The model under review builds one solid part; all positions refer to its coordinate system, in mm. A direction names the side the tool comes from. Coordinates: 2 decimals unless noted, no trailing zeros. Loops run counter-clockwise (first coordinate to the right, second up) from the corner with the lowest first, then second, coordinate; pieces in that order, holes last. Notation, with made-up numbers: M 61.25,72 L 87.25,72 A23 ccw 87.25,111 Z; hole C -39,2 d7. An arc over 180 degrees is marked long. Use CSV: the item, a comma, the result in double quotes. Start each with the question number.
from build123d import *

# Parameters (mm, degrees)
SKETCH1_R               = 15
SKETCH1_R_2             = 1
BOSS_EXTRUDE1_DEPTH     = 32.6375
SKETCH2_W               = 21.5
SKETCH2_H               = 6.35
CUT_EXTRUDE1_DEPTH      = 16
CUT_EXTRUDE1_DEPTH_BACK = 16
SKETCH3_R               = 1.5
SKETCH3_R_2             = 1
BOSS_EXTRUDE2_DEPTH     = 0.5
SKETCH4_R               = 10
SKETCH4_R_2             = 1
BOSS_EXTRUDE3_DEPTH     = 2.5
CUT_SWEEP2_PROFILE_R    = 1
SKETCH82_R              = 1.5
SKETCH82_R_2            = 1
BOSS_EXTRUDE5_DEPTH     = 0.5
SKETCH91_R              = 15
SKETCH91_R_2            = 8
CUT_EXTRUDE2_DEPTH      = 1.5
CUT_EXTRUDE2_DEPTH_BACK = 8.14375
SKETCH92_R              = 15
SKETCH92_R_2            = 10
CUT_EXTRUDE3_DEPTH      = 8.14375


with BuildPart() as part:
    # Sketch1 → Boss-Extrude1 (new body)
    with BuildSketch(Plane(origin=(0, 0, 0), x_dir=(1, 0, 0), z_dir=(0, 1, 0))):
        Circle(SKETCH1_R)
        Circle(SKETCH1_R_2, mode=Mode.SUBTRACT)
    extrude(amount=BOSS_EXTRUDE1_DEPTH)

    # Sketch2 → Cut-Extrude1 (cut, two sides)
    with BuildSketch(Plane.XY) as cut_extrude1_sk:
        with Locations((0, 16.31875)):
            Rectangle(SKETCH2_W, SKETCH2_H)
    extrude(amount=CUT_EXTRUDE1_DEPTH, mode=Mode.SUBTRACT)
    extrude(cut_extrude1_sk.sketch, amount=-CUT_EXTRUDE1_DEPTH_BACK, mode=Mode.SUBTRACT)

    # Sketch3 → Boss-Extrude2 (add)
    with BuildSketch(Plane(origin=(0, 0, 0), x_dir=(-1, 0, 0), z_dir=(0, -1, 0))):
        Circle(SKETCH3_R)
        Circle(SKETCH3_R_2, mode=Mode.SUBTRACT)
    extrude(amount=BOSS_EXTRUDE2_DEPTH)

    # Sketch4 → Boss-Extrude3 (add)
    with BuildSketch(Plane(origin=(0, 32.6375, 0), x_dir=(1, 0, 0), z_dir=(0, 1, 0))):
        Circle(SKETCH4_R)
        Circle(SKETCH4_R_2, mode=Mode.SUBTRACT)
    extrude(amount=BOSS_EXTRUDE3_DEPTH)

    # Cut-Sweep2: sweep along a path in Sketch77
    with BuildLine(Plane(origin=(0, 33.8875, 0), x_dir=(1, 0, 0), z_dir=(0, 1, 0))) as cut_sweep2_path:
        CenterArc((0, 0), 10, 0, 360)
    # Cut-Sweep2 profile (on start of the path) → Cut-Sweep2 (sweep, cut)
    with BuildSketch(Plane(origin=(10, 33.8875, 0), x_dir=(-1, 0, 0), z_dir=(0, 0, -1))):
        Circle(CUT_SWEEP2_PROFILE_R)
    sweep(path=cut_sweep2_path.line, mode=Mode.SUBTRACT)

    # Sketch82 → Boss-Extrude5 (add)
    with BuildSketch(Plane(origin=(0, 35.1375, 0), x_dir=(1, 0, 0), z_dir=(0, 1, 0))):
        Circle(SKETCH82_R)
        Circle(SKETCH82_R_2, mode=Mode.SUBTRACT)
    extrude(amount=BOSS_EXTRUDE5_DEPTH)

    # Sketch91 → Cut-Extrude2 (cut, two sides)
    with BuildSketch(Plane.XZ) as cut_extrude2_sk:
        Circle(SKETCH91_R)
        Circle(SKETCH91_R_2, mode=Mode.SUBTRACT)
    extrude(amount=CUT_EXTRUDE2_DEPTH, mode=Mode.SUBTRACT)
    extrude(cut_extrude2_sk.sketch, amount=-CUT_EXTRUDE2_DEPTH_BACK, mode=Mode.SUBTRACT)

    # Sketch92 → Cut-Extrude3 (cut)
    with BuildSketch(Plane(origin=(0, 32.6375, 0), x_dir=(1, 0, 0), z_dir=(0, 1, 0))):
        Circle(SKETCH92_R)
        Circle(SKETCH92_R_2, mode=Mode.SUBTRACT)
    extrude(amount=-CUT_EXTRUDE3_DEPTH, mode=Mode.SUBTRACT)


solid = part.part
1. Insertion check: pin 1 Ø13 at (x, z) = (-1.5, 2.5) entering from -Y; pin 2 Ø3 at (x, y) = (11.5, 11) entering from -Z; pin 3 Ø4 at (y, z) = (27.5, -2) entering from -X; pin 4 Ø8 at (x, z) = (0, 7) entering from +Y. Each pin has a flat end and moves straight along its axis. Give the tip position at first contact, or say it passes through.
2. To check wall thickness, follow line 1 along X through (y, z) = (-0.4, 0); line 2 along Y through (x, z) = (-5, -2.75); line 3 along Z through (x, y) = (0, 23.5). State the ranges of each line that lie inside material, in increasing order.
3. Add section B-B (y = 24). Write out the cut boundary in (x, z), plus the area to 3 significant figures.
4. Add section C-C (x = 0). Give the number of separate pieces and of enclosed holes in the cut face, plus the area to 3 significant figures.
5. For faces 1 (the flat face through (6, 8.144, -6)), 2 (the flat face through (-10.75, 16, 0)), 3 (the cylindrical face through (0, 27, 1)), 4 (the flat face through (3, 24.494, 10)), list the 3-axis set-ups (+Z, -Z, +X, -X, +Y, -Y) from which the entire face can be reached by the end or side of a thin tool; tool diameter is ignored.
6. Draft analysis for pull direction Y (two halves, no side actions). For faces 5 (the flat face through (2, 35.138, 0)), 6 (the cylindrical face through (-1.5, 35.38, -0.07)), 7 (the flat face through (2, 19.494, 0)), state which applies: released by +Y, released by -Y, zero draft, split by the parting line, or undercut.
7. Add section A-A (z = 11.75). Write out the cut boundary in (x, y).
Solved:
1,pin 1,"stops at y = -0.5"
1,pin 2,"stops at z = -11.18"
1,pin 3,"stops at x = -10"
1,pin 4,"stops at y = 35.14"
2,line 1,"x = -1.5 to -1, 1 to 1.5"
2,line 2,"y = 0 to 13.14, 19.49 to 35.14"
2,line 3,"z = -15 to -1, 1 to 15"
3,outline,"C 0,0 d30; hole C 0,0 d2"
3,area,"704 mm^2"
4,separate pieces,"4"
4,enclosed holes,"0"
4,area,"583 mm^2"
5,face 1,"-Y"
5,face 2,"+Z, -Z"
5,face 3,"+Y, -Y"
5,face 4,"+Y"
6,face 5,"released by +Y"
6,face 6,"zero draft"
6,face 7,"undercut"
7,outline,"M -9.32,8.14 L 9.32,8.14 L 9.32,13.14 L -9.32,13.14 Z; M -9.32,19.49 L 9.32,19.49 L 9.32,24.49 L -9.32,24.49 Z"
